Source: CAD feature listing. Evaluate the final solid. Frame: model axes, mm. A direction names the side the tool comes from. Coordinates: 2 decimals unless noted, no trailing zeros. Order: outer loops, then holes, each group sorted by start corner. A loop starts at its lowest first (then second) coordinate and runs counter-clockwise, first axis right, second up.
Autodesk Inventor part; units mm, degrees
ref_plane "YZ Plane" through (0, 0, 0) normal (1, 0, 0) x (0, 1, 0)
ref_plane "XZ Plane" through (0, 0, 0) normal (0, 1, 0) x (-1, 0, 0)
ref_plane "XY Plane" through (0, 0, 0) normal (0, 0, 1) x (1, 0, 0)
sketch "スケッチ1" plane through (0, 0, 0) normal (0, 0, 1) x (1, 0, 0)
  line L0 (-47.5, 5.75) -> (47.5, 5.75)
  line L1 (47.5, 5.75) -> (47.5, -5.75)
  line L2 (47.5, -5.75) -> (-47.5, -5.75)
  line L3 (-47.5, -5.75) -> (-47.5, 5.75)
  line L4 (-47.5, 5.75) -> (47.5, -5.75) construction
  line L5 (47.5, 5.75) -> (-47.5, -5.75) construction
  point P0 (0, 0)
  dimension "d0" = 11.5
  dimension "d1" = 95
extrude "押し出し1" add sketch "スケッチ1" along normal blind 1.5
sketch "スケッチ2" plane through (0, 0, 1.5) normal (0, 0, 1) x (1, 0, 0)
  line L0 (-42.5, 2.3) -> (42.5, 2.3)
  line L1 (42.5, 2.3) -> (42.5, -0.8)
  line L2 (42.5, -0.8) -> (-42.5, -0.8)
  line L3 (-42.5, -0.8) -> (-42.5, 2.3)
  line L4 (-47.5, -5.75) -> (47.5, -5.75)
  line L5 (47.5, -5.75) -> (47.5, 5.75)
  point P0 (0, 0)
  dimension "d8" = 3.1
  dimension "d9" = 85
  dimension "d10" = 4.95
  dimension "d11" = 5
extrude "押し出し2" cut sketch "スケッチ2" against normal blind 1.5
sketch "スケッチ3" plane through (0, 0, 1.5) normal (0, 0, 1) x (1, 0, 0)
  line L0 (-47.5, 5.75) -> (47.5, 5.75)
  line L1 (47.5, 5.75) -> (47.5, 7.25)
  line L2 (47.5, 7.25) -> (-47.5, 7.25)
  line L3 (-47.5, 7.25) -> (-47.5, 5.75)
  point P0 (0, 0)
  dimension "d14" = 95
  dimension "d15" = 1.5
extrude "押し出し3" add sketch "スケッチ3" against normal blind 21.5
sketch "スケッチ4" plane through (-47.5, 7.25, 1.5) normal (0, 1, 0) x (1, 0, 0)
  line L0 (95, 0) -> (0, 0)
  line L1 (0, 21.5) -> (95, 21.5)
  point P0 (47.5, 1.5)
  point P1 (17, 10)
  point P2 (78, 10)
  point P3 (17, 18)
  point P4 (78, 18)
  dimension "d18" = 30.5
  dimension "d19" = 30.5
  dimension "d21" = 8
  dimension "d29" = 3.5
hole "穴1" at (-30.5, 7.25, -8.5) at (30.5, 7.25, -8.5) at (-30.5, 7.25, -16.5) at (30.5, 7.25, -16.5) direction (0, -1, 0) diameter 3.1 end through all
equation "\"d27\" = Thickness"
equation "\"BendRadius\" = Thickness"
equation "\"BendReliefWidth\" = Thickness"
equation "\"BendReliefDepth\" = 0.5 * Thickness"
equation "\"CornerReliefSize\" = 4 * Thickness"
equation "\"MinimumRemnant\" = 2 * Thickness"
equation "\"TransitionRadius\" = BendRadius"
equation "\"JacobiRadiusSize\" = BendRadius"
equation "\"GapSize\" = Thickness"
properties part number "Fork 2 ver2" material "アルミニウム 5052 H32"
1. Access query for faces 4 (the face through (-1, 5.75, -10)), 5 (the face through (28.963, 6.49, -8.702)), 6 (the face through (42.5, 1, 1)). Directions: +Z, -Z, +X, -X, +Y, -Y. A direction counts if a zero-diameter tool reaches every point of the face in a straight line with its end or side. Return the directions, or none.
Findings:
face 4: -Z, +X, -X, -Y
face 5: +Y, -Y
face 6: +Z, -Z
2. Section query B-B on z = -16.5. Return loops of the section in (x, y), plus the area to 3 significant figures.
Findings:
outline: (-47.5, 5.75) - (-32.05, 5.75) - (-32.05, 7.25) - (-47.5, 7.25) - close; (-28.95, 5.75) - (28.95, 5.75) - (28.95, 7.25) - (-28.95, 7.25) - close; (32.05, 5.75) - (47.5, 5.75) - (47.5, 7.25) - (32.05, 7.25) - close
area: 133 mm2
3. Section query A-A on x = -30.5. Return loops of the section in (y, z), plus the area to 4 significant figures.
Findings:
outline: (-5.75, 0) - (-0.8, 0) - (-0.8, 1.5) - (-5.75, 1.5) - close; (2.3, 0) - (5.75, 0) - (5.75, -6.95) - (7.25, -6.95) - (7.25, 1.5) - (2.3, 1.5) - close; (5.75, -20) - (7.25, -20) - (7.25, -18.05) - (5.75, -18.05) - close; (5.75, -14.95) - (7.25, -14.95) - (7.25, -10.05) - (5.75, -10.05) - close
area: 35.55 mm2
4. Draft query along Z for faces 1 (the face through (-1, -1, 0)), 2 (the face through (-1, 2.3, 1)), 3 (the face through (-32.037, 6.49, -16.702)). Return one class per face: released by +Z, released by -Z, zero draft, split by the parting line, or undercut.
Findings:
face 1: released by -Z
face 2: zero draft
face 3: undercut
5. Ray query, line 1 (X direction, y = 6.45, z = -16.5); line 2 (Z direction, x = 30.5, y = 6.65); line 3 (Y direction, x = 42, z = -6). Return the intervals inside material, ascending.
Findings:
line 1: x = -47.5 to -32.05, -28.95 to 28.95, 32.05 to 47.5
line 2: z = -20 to -18.05, -14.95 to -10.05, -6.95 to 1.5
line 3: y = 5.75 to 7.25
6. Pin query (flat end, axial travel): P1, Ø1.5, axis at x = -3.5, z = -13.5, coming from the -Y side; P2, Ø4, axis at x = 17.5, y = 2.5, coming from the -Z side; P3, Ø5, axis at y = 4, z = -7.5, coming from the -X side; P4, Ø3, axis at x = -30.5, z = -8.5, coming from the -Y side. Return the tip coordinate at first contact, or that it passes through.
Findings:
P1: stops at y = 5.75
P2: stops at z = 0
P3: stops at x = -47.5
P4: passes through
7. Section query D-D on y = -1.75. Return loops of the section in (x, z), plus the area to 4 significant figures.
Findings:
outline: (-47.5, 0) - (47.5, 0) - (47.5, 1.5) - (-47.5, 1.5) - close
area: 142.5 mm2
8. Section query C-C on x = -17. Return loops of the section in (y, z).
Findings:
outline: (-5.75, 0) - (-0.8, 0) - (-0.8, 1.5) - (-5.75, 1.5) - close; (2.3, 0) - (5.75, 0) - (5.75, -20) - (7.25, -20) - (7.25, 1.5) - (2.3, 1.5) - close
